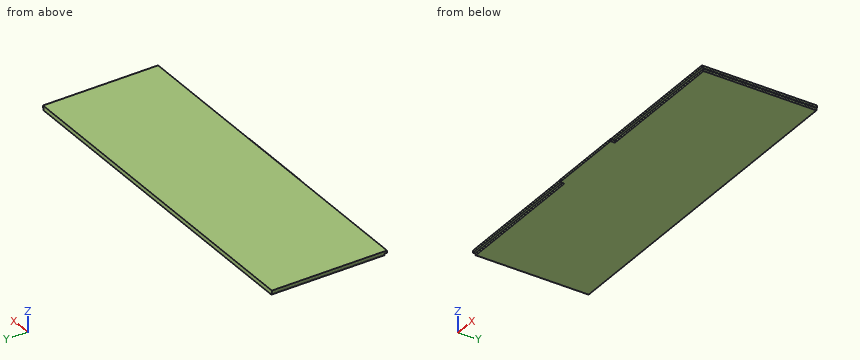
```python
from build123d import *

# Parameters (mm, degrees)
SKETCH1_W                                    = 316.5
SKETCH1_H                                    = 104.5
DIGITIZER_DEPTH                              = 2
SKETCH2_W                                    = 315
SKETCH2_H                                    = 102.5
DISPLAY_WITHOUT_MARGIN_SINCE_USING_2MM_DEPTH = 2
SKETCH3_W                                    = 70
SKETCH3_H                                    = 4
DIGITIZER_CABLE_DEPTH                        = 2


with BuildPart() as part:
    # Sketch1 → DIGITIZER (new body)
    with BuildSketch(Plane.XY):
        Rectangle(SKETCH1_W, SKETCH1_H)
    extrude(amount=DIGITIZER_DEPTH)

    # Sketch2 → DISPLAY WITHOUT MARGIN SINCE USING .2MM ADHESIVE NOW (add)
    with BuildSketch(Plane(origin=(0, 0, 0), x_dir=(-1, 0, 0), z_dir=(0, 0, -1))):
        with Locations((0, 1)):
            Rectangle(SKETCH2_W, SKETCH2_H)
    extrude(amount=DISPLAY_WITHOUT_MARGIN_SINCE_USING_2MM_DEPTH)

    # Sketch3 → DIGITIZER CABLE (add)
    with BuildSketch(Plane(origin=(0, 0, 0), x_dir=(-1, 0, 0), z_dir=(0, 0, -1))):
        with Locations((0, -52.25)):
            Rectangle(SKETCH3_W, SKETCH3_H)
    extrude(amount=DIGITIZER_CABLE_DEPTH)


solid = part.part
```
Work out the finished part from the listing and answer in its coordinate system (mm). Coordinates: 2 decimals unless noted, no trailing zeros. Loops run counter-clockwise (first coordinate to the right, second up) from the corner with the lowest first, then second, coordinate; pieces in that order, holes last. Notation, with made-up numbers: (10, 73) -> (46, 73) arc R9 cw to (46, 83) -> close; hole circle Ø6 at (43.25, 82). An arc over 180 degrees is marked (long way). Answer as CSV lines item,"result".
Q1. The part is cut by section B-B on x = 59.5. Write down the section's boundary in (y, z).
Findings:
outline,"(-52.25, 0) -> (-50.25, 0) -> (-50.25, -2) -> (52.25, -2) -> (52.25, 2) -> (-52.25, 2) -> close"
Q2. Find the intervals of material crossed by probe 1 along X at (y, z) = (19, -0.05); probe 2 along Y at (x, z) = (-78, 0.15); probe 3 along Y at (x, z) = (107, -1.35), in increasing order.
Findings:
probe 1,"x = -157.5 to 157.5"
probe 2,"y = -52.25 to 52.25"
probe 3,"y = -50.25 to 52.25"
Q3. The part is cut by section A-A on z = -0.95. Write down the section's boundary in (x, y).
Findings:
outline,"(-157.5, -50.25) -> (-35, -50.25) -> (-35, -54.25) -> (35, -54.25) -> (35, -50.25) -> (157.5, -50.25) -> (157.5, 52.25) -> (-157.5, 52.25) -> close"
Q4. Each of these flat-tipped pins is pushed along its axis until it touches: pin 1 (2 mm diameter, centred on y = -53, z = -1.5, fed in from -X); pin 2 (1 mm diameter, centred on y = -11, z = -1, fed in from +X); pin 3 (0.6 mm diameter, centred on y = -52, z = -1, fed in from +X). Where does it stop, or does it pass through?
Findings:
pin 1,"stops at x = -35"
pin 2,"stops at x = 157.5"
pin 3,"stops at x = 35"
